The listing builds one solid part. Answer for the finished solid, in the listing's coordinates (mm). A direction names the side the tool comes from. Give positions to 0.01 mm unless a question says otherwise; leave off trailing zeros. Order: outer loops, then holes, each group sorted by start corner. A loop starts at its lowest first (then second) coordinate and runs counter-clockwise, first axis right, second up.
```python
from build123d import *

# Parameters (mm, degrees)
F0_R      = 8
F1_DEPTH  = 13
F0_R_2    = 13.5
F2_DEPTH  = 3.2
F5_DEPTH  = 3
F6_W      = 27
F6_H      = 3
F7_DEPTH  = 10
F8_R      = 5
F9_R      = 5
F11_R     = 2.2611547592
F12_DEPTH = 3


with BuildPart() as f1:
    # F0 (on Front) → F1 (new body)
    with BuildSketch(Plane.XZ):
        Circle(F0_R)
    extrude(amount=F1_DEPTH)

    # F0 (on Front) → F2 (join)
    with BuildSketch(Plane.XZ):
        Circle(F0_R_2)
        Circle(F0_R, mode=Mode.SUBTRACT)
    extrude(amount=F2_DEPTH)

    # F4 (on offset) → F5 (join)
    with BuildSketch(Plane.XZ.offset(10)):
        with BuildLine():
            ThreePointArc((-4, -9.5458105994), (-2.040019644, -10.1469611141), (0, -10.35))
            ThreePointArc((0, -10.35), (2.040019644, -10.1469611141), (4, -9.5458105994))
            Line((4, -9.5458105994), (4, 9.5458105994))
            ThreePointArc((4, 9.5458105994), (2.040019644, 10.1469611141), (0, 10.35))
            ThreePointArc((0, 10.35), (-2.040019644, 10.1469611141), (-4, 9.5458105994))
            Line((-4, 9.5458105994), (-4, -9.5458105994))
        make_face()
    extrude(amount=F5_DEPTH)

    # F6 (on Front) → F7 (join)
    with BuildSketch(Plane.XZ):
        Rectangle(F6_W, F6_H)
    extrude(amount=-F7_DEPTH)

    # F8
    f8_edges = [f1.edges().sort_by_distance(p)[0] for p in [
        (-13.5, 10, 0),
    ]]
    fillet(f8_edges, radius=F8_R)

    # F9
    f9_edges = [f1.edges().sort_by_distance(p)[0] for p in [
        (13.5, 10, 0),
    ]]
    fillet(f9_edges, radius=F9_R)

    # F11 (on face) → F12 (cut, through all)
    with BuildSketch(Plane.XY.offset(1.5)):
        with Locations((0, 5)):
            Circle(F11_R)
    extrude(amount=-F12_DEPTH, mode=Mode.SUBTRACT)


solid = f1.part
```
1) Straight lines are drawn through the part: probe 1 along Y at (x, z) = (0, -0.75); probe 2 along Z at (x, y) = (-0.5, 0.5); probe 3 along Y at (x, z) = (12, -4). For each, find the intervals that lie inside material, in ascending order.
Geometry says:
probe 1: y = -13 to 2.74, 7.26 to 10
probe 2: z = -1.5 to 1.5
probe 3: y = -3.2 to 0
2) A tool of negligible diameter and unlimited length cuts with its end or side. For faces 4 (the flat face through (6, -3.2, -6)), 5 (the flat face through (3, 5, -1.5)), 6 (the flat face through (3, 5, 1.5)), 7 (the flat face through (-4, -11, -8)), from which of +Z, -Z, +X, -X, +Y, -Y can it reach the whole face along a straight path? Write none if from no direction.
Geometry says:
face 4: none
face 5: -Z, +X, -X, +Y
face 6: +Z, +X, -X, +Y
face 7: -Z, -X, -Y
3) Find section B-B (x = -0.5). Write down the section's boundary in (y, z), then the cut area to 3 significant figures.
Geometry says:
outline: (-13, -10.34) - (-10, -10.34) - (-10, -7.98) - (-3.2, -7.98) - (-3.2, -13.49) - (0, -13.49) - (0, -1.5) - (2.79, -1.5) - (2.79, 1.5) - (0, 1.5) - (0, 13.49) - (-3.2, 13.49) - (-3.2, 7.98) - (-10, 7.98) - (-10, 10.34) - (-13, 10.34) - close; (7.21, -1.5) - (10, -1.5) - (10, 1.5) - (7.21, 1.5) - close
area: 274 mm2
4) Find section A-A (y = 3.25). Write down the section's boundary in (x, z), then the cut area to 3 significant figures.
Geometry says:
outline: (-13.5, -1.5) - (-1.43, -1.5) - (-1.43, 1.5) - (-13.5, 1.5) - close; (1.43, -1.5) - (13.5, -1.5) - (13.5, 1.5) - (1.43, 1.5) - close
area: 72.4 mm2
5) Find section C-C (z = -6). Write down the section's boundary in (x, y).
Geometry says:
outline: (-12.09, -3.2) - (-5.29, -3.2) - (-5.29, -13) - (5.29, -13) - (5.29, -3.2) - (12.09, -3.2) - (12.09, 0) - (-12.09, 0) - close
6) Given P1, Ø6, axis at x = -3, z = -5.5, coming from the +Y side; P2, Ø5, axis at x = 6, y = 5.5, coming from the +Z side; P3, Ø1, axis at y = -3.5, z = 3.5, coming from the -X side; P4, Ø12, axis at x = -5.5, z = -4, coming from the +Y side, each flat-ended and moving along its own axis, determine where each tip first touches the part or whether it passes through.
Geometry says:
P1: stops at y = 0
P2: stops at z = 1.5
P3: stops at x = -13.14
P4: stops at y = 10
7) For a pull along Y with two mould halves and no side action, classify faces 1 (the flat face through (0, 0, 6)), 2 (the cylindrical face through (1.216, 6.907, 0.021)), 3 (the flat face through (-13.5, 2, 0)) as +Y half, -Y half, draft (parallel to the pull), parting line (faces both ways), or undercut.
Geometry says:
face 1: +Y half
face 2: undercut
face 3: draft
8) Find section D-D (x = -12). Write down the section's boundary in (y, z).
Geometry says:
outline: (-3.2, -6.18) - (0, -6.18) - (0, -1.5) - (8.57, -1.5) - (8.57, 1.5) - (0, 1.5) - (0, 6.18) - (-3.2, 6.18) - close
